from build123d import *

# Parameters (mm, degrees)
SKETCH1_R           = 3.551074582
BOSS_EXTRUDE1_DEPTH = 4
SKETCH2_R           = 5
BOSS_EXTRUDE2_DEPTH = 1
SKETCH3_R           = 5
BOSS_EXTRUDE3_DEPTH = 4.1


with BuildPart() as part:
    # Sketch1 → Boss-Extrude1 (new body)
    with BuildSketch(Plane(origin=(0, 0, 0), x_dir=(1, 0, 0), z_dir=(0, 1, 0))):
        with Locations(Location((0, 0, 0), (0, 0, 270))):
            Circle(SKETCH1_R)
        with BuildLine():
            ThreePointArc((-0.825, -1.428941916), (-1.166726189, -1.166726189), (-1.428941916, -0.825))
            ThreePointArc((-1.428941916, -0.825), (-1.997567148, -0.207840905), (-2.801592181, 0.0325))
            ThreePointArc((-2.801592181, 0.0325), (-2.009092181, 0.244849735), (-1.428941916, 0.825))
            ThreePointArc((-1.428941916, 0.825), (-1.159961762, 1.173451623), (-0.808423493, 1.438385017))
            ThreePointArc((-0.808423493, 1.438385017), (-0.216954174, 2.019684231), (0, 2.820106381))
            ThreePointArc((0, 2.820106381), (0.216954174, 2.019684231), (0.808423493, 1.438385017))
            ThreePointArc((0.808423493, 1.438385017), (1.159961762, 1.173451623), (1.428941916, 0.825))
            ThreePointArc((1.428941916, 0.825), (2.009092181, 0.244849735), (2.801592181, 0.0325))
            ThreePointArc((2.801592181, 0.0325), (2.03004847, -0.188087258), (1.465428549, -0.758300183))
            ThreePointArc((1.465428549, -0.758300183), (1.44756945, -0.791860269), (1.428941916, -0.825))
            ThreePointArc((1.428941916, -0.825), (1.418202031, -0.843328524), (1.407227066, -0.861517258))
            ThreePointArc((1.407227066, -0.861517258), (1.151608486, -1.181650497), (0.825, -1.428941916))
            ThreePointArc((0.825, -1.428941916), (0.244849735, -2.009092181), (0.0325, -2.801592181))
            ThreePointArc((0.0325, -2.801592181), (-0.207840905, -1.997567148), (-0.825, -1.428941916))
        make_face(mode=Mode.SUBTRACT)
    extrude(amount=BOSS_EXTRUDE1_DEPTH)

    # Sketch2 → Boss-Extrude2 (add)
    with BuildSketch(Plane(origin=(0, 4, 0), x_dir=(1, 0, 0), z_dir=(0, 1, 0))):
        with Locations(Location((0, 0, 0), (0, 0, 270))):
            Circle(SKETCH2_R)
    extrude(amount=BOSS_EXTRUDE2_DEPTH)

    # Sketch3 → Boss-Extrude3 (add)
    with BuildSketch(Plane(origin=(0, 5, 0), x_dir=(1, 0, 0), z_dir=(0, 1, 0))):
        with Locations(Location((0, 0, 0), (0, 0, 270))):
            Circle(SKETCH3_R)
        with BuildLine():
            ThreePointArc((-1.003793736, 2.880086481), (-2.156675683, 2.156675683), (-2.880086481, 1.003793736))
            ThreePointArc((-2.880086481, 1.003793736), (-3.426379172, 0.276496236), (-4.292951263, 0))
            ThreePointArc((-4.292951263, 0), (-3.426379172, -0.276496236), (-2.880086481, -1.003793736))
            ThreePointArc((-2.880086481, -1.003793736), (-2.156675683, -2.156675683), (-1.003793736, -2.880086481))
            ThreePointArc((-1.003793736, -2.880086481), (-0.276496236, -3.426379172), (0, -4.292951263))
            ThreePointArc((0, -4.292951263), (0.276496236, -3.426379172), (1.003793736, -2.880086481))
            ThreePointArc((1.003793736, -2.880086481), (2.156675683, -2.156675683), (2.880086481, -1.003793736))
            ThreePointArc((2.880086481, -1.003793736), (3.426379172, -0.276496236), (4.292951263, 0))
            ThreePointArc((4.292951263, 0), (3.426379172, 0.276496236), (2.880086481, 1.003793736))
            ThreePointArc((2.880086481, 1.003793736), (2.156675683, 2.156675683), (1.003793736, 2.880086481))
            ThreePointArc((1.003793736, 2.880086481), (0.276496236, 3.426379172), (0, 4.292951263))
            ThreePointArc((0, 4.292951263), (-0.276496236, 3.426379172), (-1.003793736, 2.880086481))
        make_face(mode=Mode.SUBTRACT)
    extrude(amount=BOSS_EXTRUDE3_DEPTH)


solid = part.part
Work out the finished part from the listing and answer in its coordinate system (mm). A direction names the side the tool comes from. Round coordinates to 2 decimals unless told otherwise and drop trailing zeros. Write each loop counter-clockwise with the first axis right and the second up, starting at its lowest first coordinate (ties: lowest second). Pieces come first, ordered by that corner, then holes. Notation, with made-up numbers: (-7, 26) - (6, 26) arc R20 ccw to (6, 35) - close; hole circle Ø11 at (14.25, -32). An arc over 180 degrees is marked (long way). Answer in a Markdown table with one row per item. Add a question column.
1. A cutting plane is placed at C-C, the plane x = -0.5. Determine the outline of the cut face in (y, z), and give its area (3 significant figures).
2. For faces 5 (the cylindrical face through (-2.17, 7.021, 2.143)), 6 (the flat face through (0, 4, 0)), determine the directions among +Z, -Z, +X, -X, +Y, -Y from which every point of the face is accessible in a straight line to the end or side of a thin tool.
3. A cutting plane is placed at B-B, the plane z = 0.5. Determine the outline of the cut face in (x, y), and give its area (3 significant figures).
4. The mould has two halves that part along X. Classify faces 1 (the flat face through (-3.3, 4, 2.2)), 2 (the cylindrical face through (0.28, 7.02, -3.42)), 3 (the cylindrical face through (-4.88, 6.51, -1.08)), 4 (the cylindrical face through (-2.143, 7.021, -2.17)): +X half, -X half, draft (parallel to the pull), parting line (faces both ways), or undercut.
5. Given pin 1 (3 mm diameter, centred on x = 0, z = -1, fed in from +Y); pin 2 (1 mm diameter, centred on x = 1.5, y = 5, fed in from -Z); pin 3 (2 mm diameter, centred on x = -3.5, y = 3.5, fed in from +Z); pin 4 (2.5 mm diameter, centred on x = -2, z = -1, fed in from +Y), each flat-ended and moving along its own axis, determine where each tip first touches the part or whether it passes through.
6. Find the intervals of material crossed by line 1 along Z through (x, y) = (-3.25, 3.5); line 2 along Z through (x, y) = (-0.5, 0.75); line 3 along X through (y, z) = (0.75, 0.25), in increasing order. Write a range as from..to.
7. A cutting plane is placed at D-D, the plane y = 8.75. Determine the outline of the cut face in (x, z), and give its area (3 significant figures).
Worked out:
| question | item | result |
|---|---|---|
| 1 | outline | (0, -3.52) - (4, -3.52) - (4, -4.97) - (9.1, -4.97) - (9.1, -3.18) - (5, -3.18) - (5, 3.18) - (9.1, 3.18) - (9.1, 4.97) - (4, 4.97) - (4, 3.52) - (0, 3.52) - (0, 1.65) - (4, 1.65) - (4, -1.66) - (0, -1.66) - close |
| 1 | area | 39.6 mm^2 |
| 2 | face 5 | +Y |
| 2 | face 6 | -Y |
| 3 | outline | (-4.97, 4) - (-3.52, 4) - (-3.52, 0) - (-1.65, 0) - (-1.65, 4) - (1.65, 4) - (1.65, 0) - (3.52, 0) - (3.52, 4) - (4.97, 4) - (4.97, 9.1) - (3.18, 9.1) - (3.18, 5) - (-3.18, 5) - (-3.18, 9.1) - (-4.97, 9.1) - close |
| 3 | area | 39.6 mm^2 |
| 4 | face 1 | draft |
| 4 | face 2 | undercut |
| 4 | face 3 | parting line |
| 4 | face 4 | undercut |
| 5 | pin 1 | y = 5 |
| 5 | pin 2 | z = -4.9 |
| 5 | pin 3 | z = 4.25 |
| 5 | pin 4 | y = 9.1 |
| 6 | line 1 | -1.43..1.43 |
| 6 | line 2 | -3.52..-1.66, 1.65..3.52 |
| 6 | line 3 | -3.54..-1.93, 1.93..3.54 |
| 7 | outline | circle Ø10 at (0, 0); hole (-4.29, 0) arc R1.5 cw to (-2.88, -1) arc R3.05 ccw to (-1, -2.88) arc R1.5 cw to (0, -4.29) arc R1.5 cw to (1, -2.88) arc R3.05 ccw to (2.88, -1) arc R1.5 cw to (4.29, 0) arc R1.5 cw to (2.88, 1) arc R3.05 ccw to (1, 2.88) arc R1.5 cw to (0, 4.29) arc R1.5 cw to (-1, 2.88) arc R3.05 ccw to (-2.88, 1) arc R1.5 cw to start |
| 7 | area | 47.2 mm^2 |
